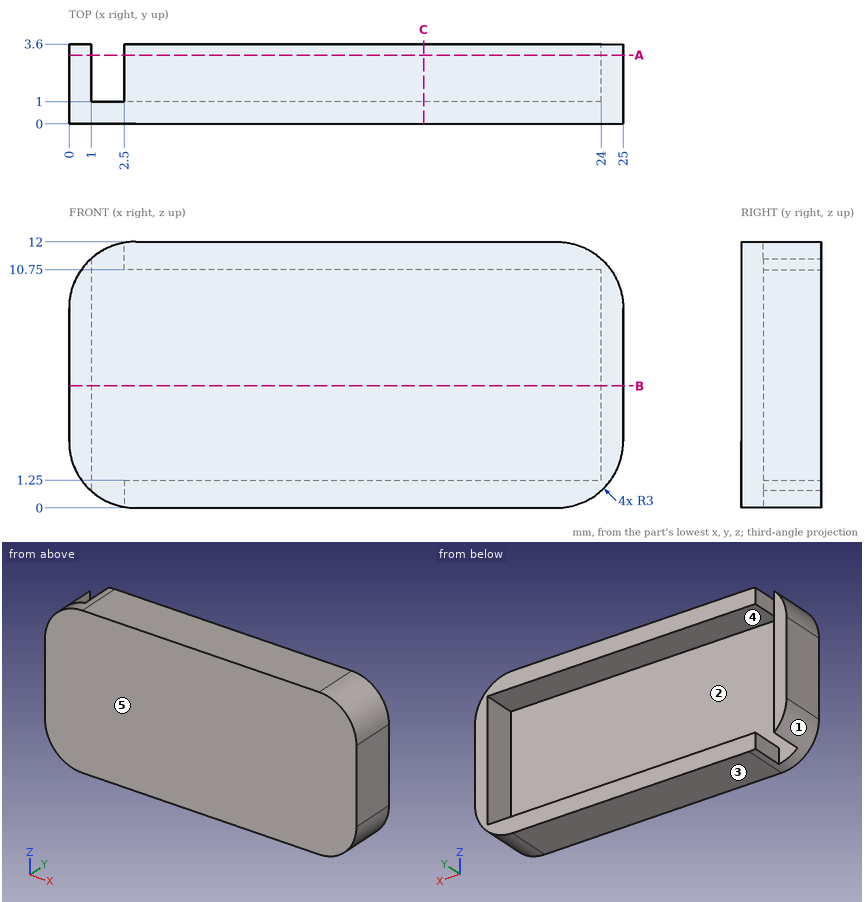
The figure shows three views and two pictorial views of one solid part (mm, origin at its lowest corner). Answer the questions. A direction names the side the tool comes from. Coordinates: 2 decimals unless noted, no trailing zeros. Loops run counter-clockwise (first coordinate to the right, second up) from the corner with the lowest first, then second, coordinate; pieces in that order, holes last.
1) Find section C-C on x = 16. Write down the section's boundary in (y, z), then the cut area to 3 significant figures.
2) Find section A-A on y = 3.1. Write down the section's boundary in (x, z), then the cut area to 3 significant figures.
3) Find section B-B on z = 5.5. Write down the section's boundary in (x, y), then the cut area to 3 significant figures.
4) A tool of negligible diameter and unlimited length cuts with its end or side. For the marked faces 4 and 5, from which of +Z, -Z, +X, -X, +Y, -Y can it reach the whole face along a straight path? Write none if from no direction.
5) Flat-ended cylindrical pins translate along their axes: pin 1 Ø5 at (x, z) = (17.5, 4) entering from -Y; pin 2 Ø0.6 at (y, z) = (2, 1) entering from -X. Find the tip coordinate at first contact, or state that the pin passes through.
6) Find the intervals of material crossed by L1, parallel to Z at x = 11.5, y = 2.1; L2, parallel to X at y = 1.65, z = 5.5; L3, parallel to Y at x = 11.25, z = 3.25, in increasing order.
7) Determine the mould class of the marked faces 1, 2 and 3 for opening direction X: pulls with the +X half, pulls with the -X half, needs draft (parallel to the pull), parting line crosses it, or undercut.
Values:
1. outline: (0, 0) - (3.6, 0) - (3.6, 1.25) - (1, 1.25) - (1, 10.75) - (3.6, 10.75) - (3.6, 12) - (0, 12) - close
1. area: 18.5 mm2
2. outline: (0, 3) arc R3 ccw to (1, 0.76) - (1, 11.24) arc R3 ccw to (0, 9) - close; (2.5, 0.04) arc R3 ccw to (3, 0) - (22, 0) arc R3 ccw to (25, 3) - (25, 9) arc R3 ccw to (22, 12) - (3, 12) arc R3 ccw to (2.5, 11.96) - (2.5, 10.75) - (24, 10.75) - (24, 1.25) - (2.5, 1.25) - close
2. area: 71.0 mm2
3. outline: (0, 0) - (25, 0) - (25, 3.6) - (24, 3.6) - (24, 1) - (1, 1) - (1, 3.6) - (0, 3.6) - close
3. area: 30.2 mm2
4. face 4: +Y
4. face 5: +Z, -Z, +X, -X, -Y
5. pin 1: stops at y = 0
5. pin 2: stops at x = 0.53
6. L1: z = 0 to 1.25, 10.75 to 12
6. L2: x = 0 to 1, 24 to 25
6. L3: y = 0 to 1
7. face 1: pulls with the -X half
7. face 2: undercut
7. face 3: needs draft
